Autodesk Inventor part; units mm, degrees
ref_plane "YZ Plane" through (0, 0, 0) normal (1, 0, 0) x (0, 1, 0)
ref_plane "XZ Plane" through (0, 0, 0) normal (0, 1, 0) x (-1, 0, 0)
ref_plane "XY Plane" through (0, 0, 0) normal (0, 0, 1) x (1, 0, 0)
sketch "axes" plane through (0, 0, 0) normal (0, 0, 1) x (1, 0, 0)
  point P0 (0, 0)
  point P1 (-35, 0)
  point P2 (0, 0)
  dimension "d0" = 35
sketch "tendon anchors" plane through (0, 0, 0) normal (0, 0, 1) x (1, 0, 0)
  line L0 (-8.2564, 0) -> (0, 0) construction
  line L1 (0, 0) -> (-7.5, -7.5) construction
  line L2 (-27.0254, 0) -> (-35, 0) construction
  line L3 (-35, 0) -> (-25.5, -5.5) construction
  dimension "d136" = 7.5
  dimension "d137" = 7.5
  dimension "d138" = 5.5
  dimension "d139" = 9.5
sketch "Sketch3" plane through (0, 0, 0) normal (0, 0, 1) x (1, 0, 0)
  line L0 (-43, 9) -> (8, 9)
  line L1 (8, 9) -> (8, -9)
  line L2 (8, -9) -> (-43, -9)
  line L3 (-43, -9) -> (-43, 9)
  point P0 (0, 0)
  point P1 (8, 0)
  point P2 (-35, 0)
  dimension "d1" = 18
  dimension "d2" = 8
  dimension "d3" = 8
extrude "base plate" add sketch "Sketch3" along normal blind 2
sketch "Sketch4" plane through (0, 0, 2) normal (0, 0, 1) x (1, 0, 0)
  line L0 (8, 9) -> (-43, 9)
  line L1 (-43, 9) -> (-43, -9)
  line L2 (-43, -9) -> (8, -9)
  line L3 (8, -9) -> (8, 9)
  line L4 (-26.5, 9) -> (-8, 9)
  line L5 (-8, 9) -> (-8, 5.4)
  line L6 (-8, 5.4) -> (-26.5, 5.4)
  line L7 (-26.5, 5.4) -> (-26.5, 9)
  line L8 (-25.5, -9) -> (-7.5, -9)
  line L9 (-7.5, -9) -> (-7.5, -4)
  line L10 (-7.5, -4) -> (-25.5, -4)
  line L11 (-25.5, -4) -> (-25.5, -9)
  point P0 (0, 0)
  point P1 (-25.5, -5.5)
  point P2 (-7.5, -7.5)
  dimension "d6" = 5
  dimension "d7" = 3.6
  dimension "d8" = 16.5
  dimension "d9" = 16
extrude "walls" add sketch "Sketch4" along normal blind 4.5 contours L5 L6 L7 L0 | L2 L11 L10 L9
sketch "Sketch5" plane through (0, 0, 2) normal (0, 0, 1) x (1, 0, 0)
  point P0 (0, 0)
  point P1 (-35, 0)
  point P2 (0, 0)
hole "joint bearings" at (-35, 0, 2) direction (0, 0, -1) diameter 3.5 end through all counterbore diameter 5 counterbore depth 1.5
fillet "front top" radius 5 1 edges at (-43, 9, 1)
fillet "front bottom" radius 8 1 edges at (-43, -9, 1)
sketch "Sketch7" plane through (0, 0, 2) normal (0, 0, 1) x (1, 0, 0)
  circle A0 centre (-35, 0) radius 4
  line L0 (-26.5, 9) -> (-38, 9)
  arc A1 (-38, 9) -> (-43, 4) centre (-38, 4) ccw
  line L1 (-26.5, 5.4) -> (-26.5, 9)
  line L2 (-38.3321, 8.989) -> (-32.1716, 2.8284)
  line L3 (-35, 0) -> (-47.831, 0) construction
  line L4 (-26.5, 5.4) -> (-34.7431, 5.4)
  point P0 (0, 0)
  dimension "d33" = 8
  dimension "d34" = 45
extrude "extension endstop" add sketch "Sketch7" along normal blind 2 contours L2 A1 L0 L1 L4
sketch "Sketch8" plane through (0, 0, 2) normal (0, 0, 1) x (1, 0, 0)
  point P0 (0, 0)
  point P1 (-35, 0)
  point P2 (-14.5, 2.5)
  point P3 (-14.5, 2.5)
  point P4 (-14.5, -1.5)
  dimension "d41" = 20.5
  dimension "d73" = 2.5
  dimension "d127" = 1.5
hole "spring pin" at (-14.5, 2.5, 2) at (-14.5, -1.5, 2) direction (0, 0, -1) diameter 1.5 end through all
sketch "Sketch10" plane through (0, 0, 2) normal (0, 0, 1) x (1, 0, 0)
  line L0 (-9, -9) -> (8, -9)
  line L1 (8, -9) -> (8, 9)
  line L2 (8, 9) -> (-9, 9)
  line L3 (-9, 9) -> (-9, -9)
  point P0 (0, 0)
  point P1 (-8, 9)
  dimension "d126" = 17
extrude "Extrusion4" add sketch "Sketch10" along normal blind 1
sketch "Sketch11" plane through (0, 0, 0) normal (0, 0, -1) x (-1, 0, 0)
  circle A0 centre (0, 0) radius 9
  line L0 (0, 9) -> (-9, 9)
  line L1 (-9, 9) -> (-9, -9)
  line L2 (-9, -9) -> (9, -9)
  line L3 (9, -9) -> (9, 0)
  dimension "d57" = 18
extrude "Extrusion5" cut sketch "Sketch11" against normal blind 1.5
fillet "Fillet5" radius 1 2 edges at (0, 9, 0.75) (-9, -9, 0.75)
fillet "Fillet6" radius 5 1 edges at (8, 9, 2.25)
fillet "Fillet7" radius 9 1 edges at (8, -9, 2.25)
sketch "Sketch12" plane through (0, 0, 3) normal (0, 0, 1) x (1, 0, 0)
  circle A0 centre (0, 0) radius 1.75
  line L0 (-0.75, -1.5811) -> (-0.75, 1.5811)
  dimension "d63" = 3.5
  dimension "d140" = 0.75
extrude "Extrusion6" cut sketch "Sketch12" against normal blind 1 contours A0 L0 picked at (0.0833, 0)
sketch "Sketch18" plane through (0, 0, 6.5) normal (0, 0, 1) x (1, 0, 0)
  line L0 (-26.5, 9) -> (-26.5, 5.4)
  line L1 (-26.5, 5.4) -> (-8, 5.4)
  line L2 (-8, 5.4) -> (-8, 9)
  line L3 (-8, 9) -> (-26.5, 9)
  line L4 (-25.5, -9) -> (-7.5, -9)
  line L5 (-7.5, -9) -> (-7.5, -4)
  line L6 (-7.5, -4) -> (-25.5, -4)
  line L7 (-25.5, -4) -> (-25.5, -9)
  circle A0 centre (-14.5, 2.5) radius 0.75
  line L8 (-16.5, 5.4) -> (-12.5, 5.4)
  line L9 (-12.5, 5.4) -> (-12.5, -4)
  line L10 (-12.5, -4) -> (-16.5, -4)
  line L11 (-16.5, -4) -> (-16.5, 5.4)
  line L12 (-14.5, 2.5) -> (-14.5, -2.026) construction
  point P0 (0, 0)
  dimension "d105" = 4
extrude "Extrusion8" add sketch "Sketch18" along normal blind 1.5 contours L3 L2 L1 L0 | L1 L9 L6 L11 | L6 L5 L4 L7 | A0
sketch "Sketch19" plane through (0, 0, 6.5) normal (0, 0, -1) x (-1, 0, 0)
  circle A0 centre (14.5, 2.5) radius 0.75
  circle A1 centre (14.5, -1.5) radius 0.75
  point P0 (0, 0)
hole "spring pins support" at (-14.5, 2.5, 6.5) at (-14.5, -1.5, 6.5) direction (0, 0, 1) diameter 1 end through all counterbore diameter 1.5 counterbore depth 1.25
sketch "Sketch14" plane through (0, 0, 3) normal (0, 0, 1) x (1, 0, 0)
  line L0 (-0.75, -1.5811) -> (-0.75, 1.5811)
  arc A0 (-0.75, -1) -> (-0.75, 1) centre (0, 0) ccw
  dimension "d133" = 2.5
extrude "Extrusion11" cut sketch "Sketch14" against normal through all
sketch "Sketch17" plane through (0, 0, 8) normal (0, 0, 1) x (1, 0, 0)
  point P0 (5, 0)
  point P1 (-21, -7)
  point P2 (-13, -7)
  point P3 (-24.5, 7)
  point P4 (-10.5, 7)
  point P5 (-35, 0)
  point P6 (0, 0)
  point P7 (-35, 0)
  point P8 (0, 0)
  dimension "d92" = 7
  dimension "d93" = 7
  dimension "d94" = 10.5
  dimension "d95" = 10.5
  dimension "d96" = 14
  dimension "d97" = 13
hole "mounting" at (-24.5, 7, 8) at (-10.5, 7, 8) at (-21, -7, 8) at (-13, -7, 8) direction (0, 0, -1) diameter 1.6 depth 6 tip angle 118
sketch "Sketch20" plane through (-43, 4, 0) normal (-1, 0, 0) x (0, 0, 1)
  line L0 (3, 5) -> (20, 5)
  line L1 (20, 5) -> (20, -13)
  line L2 (20, -13) -> (3, -13)
  line L3 (0, -10) -> (0, 2)
  arc A0 (3, 5) -> (0, 2) centre (3, 2) ccw
  arc A1 (0, -10) -> (3, -13) centre (3, -10) ccw
  point P0 (0, -4)
  point P1 (0, 5)
  point P2 (0, -13)
  point P3 (0, -13)
  dimension "d115" = 20
  dimension "d116" = 3
extrude "side fillet" cut sketch "Sketch20" against normal through all keep common part
fillet "Fillet8" radius 1 5 edges at (-39.0048, -7.9255, 0.6994) (-43, 1.5, 0) (-42.8945, 5.0215, 0) (-41.0629, 7.9521, 0.722) (-42.5485, -3.6495, 0)
sketch "Sketch21" plane through (-38, 9, 4) normal (0, 1, 0) x (1, 0, 0)
  line L0 (11.5, 0) -> (0, 0)
  line L1 (11.5, 0) -> (11.5, -4)
  line L2 (10, -4) -> (10, -4) construction
  line L3 (11.15, -4) -> (11.15, -4)
  line L4 (8.85, -4) -> (8.85, -4)
  arc A0 (8.85, -4) -> (11.15, -4) centre (10, -4) ccw
  arc A1 (11.15, -4) -> (8.85, -4) centre (10, -4) ccw
  line L5 (8.85, -4) -> (7.85, -4)
  line L6 (7.85, -4) -> (7.85, 0)
  line L7 (11.15, -4) -> (11.5, -4)
  point P0 (38, 4)
  point P1 (10, -3.75)
  point P2 (3, 4)
  dimension "d120" = 2.3
  dimension "d121" = 7
  dimension "d122" = 0
  dimension "d123" = 1
extrude "cable clip" add sketch "Sketch21" against normal blind 3 contours L1 L7 A1 L5 L6 L0
chamfer "Chamfer1" distance 1 angle 45 3 edges at (-9, 0.7, 2) (-21.8716, 5.4, 2) (-17.25, -4, 2)
fillet "Fillet9" radius 1 4 edges at (-16.5, 5.4, 7.25) (-12.5, 5.4, 7.25) (-12.5, -4, 7.25) (-16.5, -4, 7.25)
fillet "Fillet10" radius 1 4 edges at (-17, -4, 6.5) (-12, -4, 6.5) (-12, 5.4, 6.5) (-17, 5.4, 6.5)
equation "\"MCP_PIP_length\" = F5_MCP_PIP_length"
equation "\"PIP_spring_length\" = F5_PIP_spring_length"
properties part number "phalanx 1 R F5"
Read the model definition and answer for the solid it produces. Units are mm, in the model's axes. A direction names the side the tool comes from. Give positions to 0.01 mm unless a question says otherwise; leave off trailing zeros. Write each loop counter-clockwise with the first axis right and the second up, starting at its lowest first coordinate (ties: lowest second). Pieces come first, ordered by that corner, then holes. Notation, with made-up numbers: (2.5, -12) - (44.5, -12) arc R28 cw to (44.5, 23) - close; hole circle Ø10 at (6, -33.75). An arc over 180 degrees is marked (long way). Use CSV: the item, a comma, the result in double quotes. Start each with the question number.
(1) For faces 4 (the flat face through (-22.1, 4.9, 2.5)), 5 (the flat face through (1, -1, 2)), 6 (the cylindrical face through (-15.244, 2.598, 0.986)), determine the directions among +Z, -Z, +X, -X, +Y, -Y from which every point of the face is accessible in a straight line to the end or side of a thin tool.
(2) Determine the mould class of faces 1 (the flat face through (-9, -4, 1)), 2 (the cylindrical face through (-42.48, 6.22, 1.49)), 3 (the flat face through (-17.4, -3.5, 2.5)) for opening direction Y: +Y half, -Y half, draft (parallel to the pull), parting line (faces both ways), or undercut.
(3) Find section A-A (x = -28). Give the vertices of the cut face in (y, z).
(4) Find section B-B (x = -14.5). Count the separate pieces of the cut face and the enclosed holes in it, plus the area to 3 significant figures.
(5) Find section C-C (x = 3.5). Give the vertices of the cut face in (y, z).
(6) Consider line 1 along Y through (x, z) = (-10.5, 6.8); line 2 along Y through (x, z) = (-14.5, 7.95); line 3 along X through (y, z) = (-7, 6.8). Determine where each line is inside the solid, lowest interval first.
(7) Given P1, Ø1.1, axis at y = 8, z = 6, coming from the +X side; P2, Ø1.5, axis at x = -36, y = -0.5, coming from the +Z side; P3, Ø2, axis at y = -3, z = 2, coming from the +X side; P4, Ø2.5, axis at x = -13, y = -7, coming from the +Z side, each flat-ended and moving along its own axis, determine where each tip first touches the part or whether it passes through.
Findings below:
1,face 4,"-X"
1,face 5,"+Z"
1,face 6,"-Z"
2,face 1,"draft"
2,face 2,"+Y half"
2,face 3,"undercut"
3,outline,"(-8.83, 2) arc R3 ccw to (-6, 0) - (6, 0) arc R3 ccw to (9, 3) - (9, 6.85) - (6, 6.85) - (6, 4) - (5.4, 4) - (5.4, 3) - (4.4, 2) - close"
4,separate pieces,"4"
4,enclosed holes,"0"
4,area,"89.0 mm2"
5,outline,"(-7.79, 1.5) - (8.6, 1.5) arc R3 ccw to (8.97, 2.61) - (8.97, 3) - (-7.79, 3) - close"
6,line 1,"-9 to -4, 5.4 to 6.2, 7.8 to 9"
6,line 2,"-9 to -2, -1 to 2, 3 to 9"
6,line 3,"-25.5 to -21.8, -20.2 to -13.8, -12.2 to -7.5"
7,P1,"x = -8"
7,P2,"z = 0.5"
7,P3,"x = 7.77"
7,P4,"z = 8"
